Check sheet for the drawn part. Datum: minimum x, y, z corner. Units: mm. Round coordinates to 2 decimals unless told otherwise and drop trailing zeros. Loops run counter-clockwise (first coordinate to the right, second up) from the corner with the lowest first, then second, coordinate; pieces in that order, holes last.
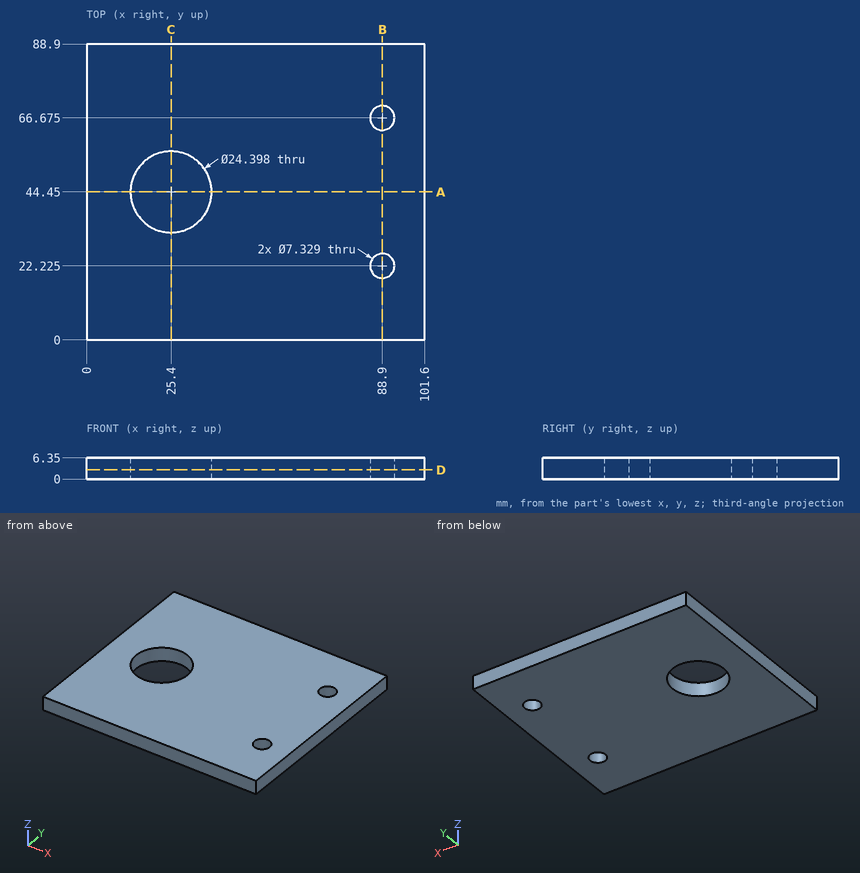
1. Section check B-B (x = 88.9). Enter the section's corners in (y, z).
2. Section check A-A (y = 44.45). Enter the section's corners in (x, z), then the cut area to 3 significant figures.
3. Scan lines: L1, parallel to Y at x = 88.9, z = 4.5; L2, parallel to X at y = 45, z = 3.25; L3, parallel to X at y = 23, z = 2.5. Record each from-to range of solid material in increasing order.
4. Section check D-D (z = 2.75). Give the number of separate pieces and of enclosed holes in the cut face, then the cut area to 3 significant figures.
5. Section check C-C (x = 25.4). Enter the section's corners in (y, z).
Taken from the geometry:
1. outline: (0, 0) - (18.56, 0) - (18.56, 6.35) - (0, 6.35) - close; (25.89, 0) - (63.01, 0) - (63.01, 6.35) - (25.89, 6.35) - close; (70.34, 0) - (88.9, 0) - (88.9, 6.35) - (70.34, 6.35) - close
2. outline: (0, 0) - (13.2, 0) - (13.2, 6.35) - (0, 6.35) - close; (37.6, 0) - (101.6, 0) - (101.6, 6.35) - (37.6, 6.35) - close
2. area: 490 mm2
3. L1: y = 0 to 18.56, 25.89 to 63.01, 70.34 to 88.9
3. L2: x = 0 to 13.21, 37.59 to 101.6
3. L3: x = 0 to 85.32, 92.48 to 101.6
4. separate pieces: 1
4. enclosed holes: 3
4. area: 8,480 mm2
5. outline: (0, 0) - (32.25, 0) - (32.25, 6.35) - (0, 6.35) - close; (56.65, 0) - (88.9, 0) - (88.9, 6.35) - (56.65, 6.35) - close
